```python
from build123d import *

# Parameters (mm, degrees)
SKETCH1_W            = 50
SKETCH1_H            = 150
SKETCH1_R            = 2.5
BOSS_EXTRUDE1_DEPTH  = 15
BOSS_EXTRUDE2_DEPTH  = 90
SKETCH3_W            = 250
SKETCH3_H            = 15
BOSS_EXTRUDE3_DEPTH  = 150
BOSS_EXTRUDE8_DEPTH  = 10
CUT_EXTRUDE1_DEPTH   = 10
SKETCH10_W           = 115
SKETCH10_H           = 165
BOSS_EXTRUDE12_DEPTH = 15
CUT_EXTRUDE3_DEPTH   = 181
SKETCH13_R           = 2.5
CUT_EXTRUDE4_DEPTH   = 116.470053838
SKETCH14_R           = 2.5
CUT_EXTRUDE5_DEPTH   = 181


with BuildPart() as part:
    # Sketch1 → Boss-Extrude1 (new body)
    with BuildSketch(Plane(origin=(0, 0, 0), x_dir=(1, 0, 0), z_dir=(0, 1, 0))):
        Polygon((0, 90), (0, 75), (50, 75), (50, -75), (0, -75), (0, -90), (250, -90), (250, 90), align=None)
        with Locations((25, 0)):
            Rectangle(SKETCH1_W, SKETCH1_H)
        with Locations((7.5, -67.5)):
            Circle(SKETCH1_R, mode=Mode.SUBTRACT)
        with Locations((42.5, -67.5)):
            Circle(SKETCH1_R, mode=Mode.SUBTRACT)
        with Locations((7.5, 67.5)):
            Circle(SKETCH1_R, mode=Mode.SUBTRACT)
        with Locations((42.5, 67.5)):
            Circle(SKETCH1_R, mode=Mode.SUBTRACT)
    extrude(amount=BOSS_EXTRUDE1_DEPTH)

    # Sketch2 → Boss-Extrude2 (add, symmetric)
    with BuildSketch(Plane.XY):
        Polygon((0, 0), (-200, -115.470053838), (-200, -100.470053838), (0, 15), align=None)
    extrude(amount=BOSS_EXTRUDE2_DEPTH, both=True)

    # Sketch3 → Boss-Extrude3 (add)
    with BuildSketch(Plane(origin=(0, 15, 0), x_dir=(1, 0, 0), z_dir=(0, 1, 0))):
        with Locations((125, 82.5)):
            Rectangle(SKETCH3_W, SKETCH3_H)
        with Locations((125, -82.5)):
            Rectangle(SKETCH3_W, SKETCH3_H)
    extrude(amount=BOSS_EXTRUDE3_DEPTH)

    # Sketch8 → Boss-Extrude8 (add)
    with BuildSketch(Plane.XY.offset(90)):
        Polygon((0, 15), (-200, -100.470053838), (-200, 49.529946162), (0, 165), align=None)
    boss_extrude8 = extrude(amount=-BOSS_EXTRUDE8_DEPTH)

    # Mirror1: Boss-Extrude8 across plane
    add(boss_extrude8.mirror(Plane.XY))

    # Sketch9 → Cut-Extrude1 (cut)
    with BuildSketch(Plane.XY.offset(-75)):
        with BuildLine():
            Line((-190, 12.520327219), (-190, -87.479672781))
            ThreePointArc((-190, -87.479672781), (-192.5, -89.979672781), (-195, -87.479672781))
            Line((-195, -87.479672781), (-195, 12.520327219))
            ThreePointArc((-195, 12.520327219), (-192.5, 15.020327219), (-190, 12.520327219))
        make_face()
    cut_extrude1 = extrude(amount=-CUT_EXTRUDE1_DEPTH, mode=Mode.SUBTRACT)

    # Mirror2: Cut-Extrude1 across plane
    add(cut_extrude1.mirror(Plane.XY), mode=Mode.SUBTRACT)

    # Sketch10 → Boss-Extrude12 (add)
    with BuildSketch(Plane(origin=(250, 0, 0), x_dir=(0, 0, -1), z_dir=(1, 0, 0))):
        with Locations((-32.5, 82.5)):
            Rectangle(SKETCH10_W, SKETCH10_H)
    boss_extrude12 = extrude(amount=-BOSS_EXTRUDE12_DEPTH)

    # Mirror3: Boss-Extrude12 across plane
    add(boss_extrude12.mirror(Plane.XY))

    # Sketch12 → Cut-Extrude3 (cut, through all)
    with BuildSketch(Plane.XY.offset(90)):
        Polygon((0, 165), (250, 165), (250, 0), (0, 0), (-49.62663195, 136.348050685), align=None)
    extrude(amount=-CUT_EXTRUDE3_DEPTH, mode=Mode.SUBTRACT)

    # Sketch13 → Cut-Extrude4 (cut, through all)
    with BuildSketch(Plane(origin=(0, 0, 0), x_dir=(1, 0, 0), z_dir=(0, 1, 0))):
        with Locations((-142.5, 67.5)):
            Circle(SKETCH13_R)
        with Locations((-107.5, 67.5)):
            Circle(SKETCH13_R)
        with Locations((-142.5, -67.5)):
            Circle(SKETCH13_R)
        with Locations((-107.5, -67.5)):
            Circle(SKETCH13_R)
    extrude(amount=-CUT_EXTRUDE4_DEPTH, mode=Mode.SUBTRACT)

    # Sketch14 → Cut-Extrude5 (cut, through all)
    with BuildSketch(Plane(origin=(0, 0, -90), x_dir=(-1, 0, 0), z_dir=(0, 0, -1))):
        with Locations((95, 11.348050685)):
            Circle(SKETCH14_R)
        with Locations((130, 11.348050685)):
            Circle(SKETCH14_R)
        with Locations((95, 26.348050685)):
            Circle(SKETCH14_R)
        with Locations((130, 26.348050685)):
            Circle(SKETCH14_R)
    extrude(amount=-CUT_EXTRUDE5_DEPTH, mode=Mode.SUBTRACT)


solid = part.part
```
Check sheet for the modelled part. Datum: model origin and axes. Units: mm. A direction names the side the tool comes from. Round coordinates to 2 decimals unless told otherwise and drop trailing zeros. Write each loop counter-clockwise with the first axis right and the second up, starting at its lowest first coordinate (ties: lowest second). Pieces come first, ordered by that corner, then holes. Notation, with made-up numbers: (34, 1) -> (93, 1) arc R20 ccw to (93, 20) -> close; hole circle Ø8 at (46, 58.25). An arc over 180 degrees is marked (long way). Put each result on its own line as item: value.
(1) Sectioned sample at D-D (z = -33). Enter the section's corners in (x, y).
Values found:
outline: (-200, -115.47) -> (0, 0) -> (-4.51, 12.4) -> (-200, -100.47) -> close
(2) Tool access check on faces 1 (the face through (-125.87, 92.33, -85.07)), 2 (the face through (-103.624, -44.827, 1.12)). Record the directions out of +Z, -Z, +X, -X, +Y, -Y that give a thin tool (end or side, any length) a straight path to the whole face; none if there is none.
Values found:
face 1: +Z, -Z, -X, +Y
face 2: -X, +Y
(3) Sectioned sample at A-A (y = 35). Enter the section's corners in (x, z).
Values found:
outline: (-200, -90) -> (-12.74, -90) -> (-12.74, -80) -> (-200, -80) -> close; (-200, 80) -> (-12.74, 80) -> (-12.74, 90) -> (-200, 90) -> close
(4) Material ranges on line 1 (Z direction, x = -155.5, y = 51); line 2 (Y direction, x = -95, z = 83); line 3 (Z direction, x = -191, y = -61), recorded low to high.
Values found:
line 1: z = -90 to -80, 80 to 90
line 2: y = -54.85 to 8.85, 13.85 to 23.85, 28.85 to 110.15
line 3: z = -90 to -85, 85 to 90
(5) Sectioned sample at C-C (y = -15). Enter the section's corners in (x, z), plus the area to 3 significant figures.
Values found:
outline: (-200, -90) -> (-25.98, -90) -> (-25.98, 90) -> (-200, 90) -> (-200, 80) -> (-195, 80) -> (-195, 85) -> (-190, 85) -> (-190, 80) -> (-51.96, 80) -> (-51.96, -80) -> (-190, -80) -> (-190, -85) -> (-195, -85) -> (-195, -80) -> (-200, -80) -> close
area: 7,590 mm^2
(6) Go/stop test with flat-tipped pins: pin 1 Ø8 at (y, z) = (-60.5, 50) entering from -X; pin 2 Ø6 at (x, z) = (-135.5, -29) entering from -Y; pin 3 Ø4 at (y, z) = (9, -29.5) entering from -X. Record where each tip stops, or that it passes through.
Values found:
pin 1: stops at x = -137.7
pin 2: stops at y = -79.96
pin 3: stops at x = -13.86
(7) Sectioned sample at B-B (x = -86). Enter the section's corners in (y, z).
Values found:
outline: (-49.65, -90) -> (115.35, -90) -> (115.35, -80) -> (-34.65, -80) -> (-34.65, 80) -> (115.35, 80) -> (115.35, 90) -> (-49.65, 90) -> close
(8) Mould release check, pull along Z, two halves, no side actions. Record for faces 3 (the face through (-2.641, 7.257, 13.753)), 4 (the face through (-121, 12, 90)), 5 (the face through (-123, 20, 80)): released by +Z, released by -Z, zero draft, split by the parting line, or undercut.
Values found:
face 3: zero draft
face 4: released by +Z
face 5: undercut
